Here's how the part is built. I have some questions about the finished solid (model axes, mm). A direction names the side the tool comes from. Round coordinates to 2 decimals unless told otherwise and drop trailing zeros. Loops run counter-clockwise (first coordinate to the right, second up) from the corner with the lowest first, then second, coordinate; pieces in that order, holes last. Notation, with made-up numbers: (-40, -8.5) -> (-12, -8.5) arc R19 ccw to (-12, 4.5) -> close; hole circle Ø10 at (14.5, 48.5). An arc over 180 degrees is marked (long way). Use CSV: the item, a comma, the result in double quotes. Start each with the question number.
from build123d import *

# Parameters (mm, degrees)
SKETCH2_R           = 15
BOSS_EXTRUDE1_DEPTH = 12
SHELL1_T            = -2
SKETCH4_R           = 2.75
CUT_EXTRUDE1_DEPTH  = 25.372115214
SKETCH5_R           = 17
SKETCH5_R_2         = 15
BOSS_EXTRUDE3_DEPTH = 2
BOSS_EXTRUDE5_START = 4
SKETCH7_R           = 4.25
SKETCH7_R_2         = 2.75
BOSS_EXTRUDE5_DEPTH = 4
SKETCH6_R           = 6.25
SKETCH6_R_2         = 2.75
BOSS_EXTRUDE4_DEPTH = 1.5


with BuildPart() as part:
    # Sketch2 → Boss-Extrude1 (new body)
    with BuildSketch(Plane(origin=(0, 0, 0), x_dir=(1, 0, 0), z_dir=(0, 1, 0))):
        with Locations(Location((0, 0, 0), (0, 0, 270))):
            Circle(SKETCH2_R)
    extrude(amount=BOSS_EXTRUDE1_DEPTH)

    # Shell1
    shell1_openings = [part.faces().sort_by_distance(p)[0] for p in [
        (0, 12, 0),
    ]]
    offset(amount=SHELL1_T, openings=shell1_openings, kind=Kind.INTERSECTION)

    # Sketch4 → Cut-Extrude1 (cut, through all)
    with BuildSketch(Plane.XZ):
        with Locations(Location((0, 0, 0), (0, 0, 270))):
            Circle(SKETCH4_R)
    extrude(amount=-CUT_EXTRUDE1_DEPTH, mode=Mode.SUBTRACT)

    # Sketch5 → Boss-Extrude3 (add)
    with BuildSketch(Plane.XZ):
        with Locations(Location((0, 0, 0), (0, 0, 270))):
            Circle(SKETCH5_R)
        with Locations(Location((0, 0, 0), (0, 0, 270))):
            Circle(SKETCH5_R_2, mode=Mode.SUBTRACT)
    extrude(amount=-BOSS_EXTRUDE3_DEPTH)

    # Sketch7 → Boss-Extrude5 (add)
    with BuildSketch(Plane.XZ.offset(BOSS_EXTRUDE5_START)):
        with Locations(Location((0, 0, 0), (0, 0, 90))):
            Circle(SKETCH7_R)
        with Locations(Location((0, 0, 0), (0, 0, 270))):
            Circle(SKETCH7_R_2, mode=Mode.SUBTRACT)
    extrude(amount=-BOSS_EXTRUDE5_DEPTH)

    # Sketch6 → Boss-Extrude4 (add)
    with BuildSketch(Plane(origin=(0, 2, 0), x_dir=(1, 0, 0), z_dir=(0, 1, 0))):
        with Locations(Location((0, 0, 0), (0, 0, 90))):
            Circle(SKETCH6_R)
        with Locations(Location((0, 0, 0), (0, 0, 90))):
            Circle(SKETCH6_R_2, mode=Mode.SUBTRACT)
    extrude(amount=BOSS_EXTRUDE4_DEPTH)


solid = part.part
Q1. I want a section at A-A, the plane x = 0. List the corners of the cut face in (y, z) for me, then the cut area to 4 significant figures.
Q2. I need wall thicknesses on line 1 along X through (y, z) = (2.25, 0); line 2 along Z through (x, y) = (0, 6.75). Which ranges of each line are inside material? Lowest first, please.
Q3. For faces 1 (the flat face through (3, -4, 0)), 2 (the flat face through (-4, 0, -4)), 3 (the cylindrical face through (0.66, 6.93, -14.985)), which set-ups out of +Z, -Z, +X, -X, +Y, -Y let a thin tool reach every point of the face, with its end or its side?
Q4. I want a section at C-C, the plane y = -2.25. List the corners of the cut face in (x, z) for me, then the cut area to 3 significant figures.
Q5. If we mould it in two halves opening along Z, with no side actions, what happens to faces 4 (the flat face through (-14, 2, -6)), 5 (the cylindrical face through (2.685, -0.303, 0.596)), 6 (the cylindrical face through (16.855, 0.986, 2.213))? For each: pulls with the +Z half, pulls with the -Z half, needs draft (parallel to the pull), parting line crosses it, or undercut.
Q6. Will these pins go through, and if not, where does the flat tip stop? pin 1 Ø14 at (x, z) = (2.5, 1) entering from +Y; pin 2 Ø4 at (y, z) = (8, 3) entering from -X; pin 3 Ø4 at (x, z) = (6, -8) entering from -Y.
Q7. I want a section at D-D, the plane x = 12. List the corners of the cut face in (y, z) for me, then the cut area to 3 significant figures.
Q8. I want a section at B-B, the plane z = 0. List the corners of the cut face in (x, y) for me.
Values found:
1,outline,"(-4, -4.25) -> (0, -4.25) -> (0, -17) -> (2, -17) -> (2, -15) -> (12, -15) -> (12, -13) -> (2, -13) -> (2, -6.25) -> (3.5, -6.25) -> (3.5, -2.75) -> (-4, -2.75) -> close; (-4, 2.75) -> (3.5, 2.75) -> (3.5, 6.25) -> (2, 6.25) -> (2, 13) -> (12, 13) -> (12, 15) -> (2, 15) -> (2, 17) -> (0, 17) -> (0, 4.25) -> (-4, 4.25) -> close"
1,area,"119.5 mm2"
2,line 1,"-15 to -13, -6.25 to -2.75, 2.75 to 6.25, 13 to 15"
2,line 2,"-15 to -13, 13 to 15"
3,face 1,"+Z, -Z, +X, -X, -Y"
3,face 2,"-Y"
3,face 3,"+Y"
4,outline,"circle Ø8.5 at (0, 0); hole circle Ø5.5 at (0, 0)"
4,area,"33.0 mm2"
5,face 4,"needs draft"
5,face 5,"undercut"
5,face 6,"parting line crosses it"
6,pin 1,"y = 3.5"
6,pin 2,"x = -14.97"
6,pin 3,"y = 0"
7,outline,"(0, -12.04) -> (2, -12.04) -> (2, -9) -> (12, -9) -> (12, -5) -> (2, -5) -> (2, 5) -> (12, 5) -> (12, 9) -> (2, 9) -> (2, 12.04) -> (0, 12.04) -> close"
7,area,"128 mm2"
8,outline,"(-17, 0) -> (-4.25, 0) -> (-4.25, -4) -> (-2.75, -4) -> (-2.75, 3.5) -> (-6.25, 3.5) -> (-6.25, 2) -> (-13, 2) -> (-13, 12) -> (-15, 12) -> (-15, 2) -> (-17, 2) -> close; (2.75, -4) -> (4.25, -4) -> (4.25, 0) -> (17, 0) -> (17, 2) -> (15, 2) -> (15, 12) -> (13, 12) -> (13, 2) -> (6.25, 2) -> (6.25, 3.5) -> (2.75, 3.5) -> close"
